Design review of the part built by this model. Coordinates are the model's own, in mm. Face numbers are marked on the shaded views. A direction names the side the tool comes from. Round coordinates to 2 decimals unless told otherwise and drop trailing zeros. Loops run counter-clockwise (first coordinate to the right, second up) from the corner with the lowest first, then second, coordinate; pieces in that order, holes last. Notation, with made-up numbers: M -23.5,25.25 L -2.5,25.25 A12 ccw -2.5,34.25 Z; hole C 86.25,80 d9. An arc over 180 degrees is marked long. One line per item, written item: value. Start each with the question number.
Item 1: For line 1 along Y through (x, z) = (-7, 2.4) (3 decimals); line 2 along Y through (x, z) = (12, 2.35); line 3 along Y through (x, z) = (-3, 2.8), list the stretches that pass through material, from the lowest coordinate up.
Item 2: For the marked faces 1, 2 and 3, list the 3-axis set-ups (+Z, -Z, +X, -X, +Y, -Y) from which the entire face can be reached by the end or side of a thin tool; tool diameter is ignored.
Item 3: Mouldability with a two-part tool opening along Y and no side actions: class the marked faces 4, 5, 6 and 7 as released by +Y, released by -Y, zero draft, split by the parting line, or undercut.
Item 4: We need section D-D (z = 2.55). State how many separate pieces and enclosed holes the cut face has, then the cut area to 3 significant figures.
Item 5: We need section A-A (x = -1.25). Write out the cut boundary in (y, z), then the cut area to 3 significant figures.
Item 6: Clearance check with flat-ended pins moving along their axes: pin 1 (1.5 mm diameter, centred on x = 2.5, z = 2, fed in from +Y); pin 2 (0.9 mm diameter, centred on y = 5, z = 1.5, fed in from -X); pin 3 (0.9 mm diameter, centred on x = -4, z = 1.5, fed in from -Y). State where each tip first meets the part, or that it passes through.
Item 7: We need section B-B (x = 11.5). Write out the cut boundary in (y, z), then the cut area to 3 significant figures.
Item 8: We need section C-C (x = -6). Write out the cut boundary in (y, z).
from build123d import *

# Parameters (mm, degrees)
BOSS_EXTRUDE1_DEPTH  = 3
SKETCH2_W            = 8
SKETCH2_H            = 3
BOSS_EXTRUDE2_DEPTH  = 7
SKETCH3_W            = 8
SKETCH3_H            = 3
BOSS_EXTRUDE3_DEPTH  = 7
SKETCH4_R            = 3.300094696
BOSS_EXTRUDE4_DEPTH  = 0.5
SKETCH5_R            = 3.300094696
BOSS_EXTRUDE5_DEPTH  = 0.5
CUT_EXTRUDE1_DEPTH   = 4
M3_CLEARANCE_HOLE2_D = 3.4
M3_CLEARANCE_HOLE1_D = 3.4
FILLET1_R            = 0.5
FILLET2_R            = 2
FILLET3_R            = 3


with BuildPart() as part:
    # Sketch1 → Boss-Extrude1 (new body)
    with BuildSketch(Plane(origin=(0, 0, 0), x_dir=(-1, 0, 0), z_dir=(0, 0, -1))):
        with BuildLine():
            Line((-16, 3), (-16, -3))
            Line((-16, -3), (9.864129683, -3))
            ThreePointArc((9.864129683, -3), (9.35323266, -6.252551424), (8.487341847, -9.429080919))
            ThreePointArc((8.487341847, -9.429080919), (3.884055388, -13.461974782), (9.996965881, -13.756600705))
            ThreePointArc((9.996965881, -13.756600705), (13.015220034, 0), (9.996965881, 13.756600705))
            ThreePointArc((9.996965881, 13.756600705), (3.884055388, 13.461974781), (8.487341847, 9.429080919))
            ThreePointArc((8.487341847, 9.429080919), (9.35323266, 6.252551424), (9.864129683, 3))
            Line((9.864129683, 3), (-16, 3))
        make_face()
    extrude(amount=-BOSS_EXTRUDE1_DEPTH)

    # Sketch2 → Boss-Extrude2 (add)
    with BuildSketch(Plane.XZ.offset(3)):
        with Locations((12, 1.5)):
            Rectangle(SKETCH2_W, SKETCH2_H)
    extrude(amount=BOSS_EXTRUDE2_DEPTH)

    # Sketch3 → Boss-Extrude3 (add)
    with BuildSketch(Plane(origin=(0, 3, 0), x_dir=(-1, 0, 0), z_dir=(0, 1, 0))):
        with Locations((-12, 1.5)):
            Rectangle(SKETCH3_W, SKETCH3_H)
    extrude(amount=BOSS_EXTRUDE3_DEPTH)

    # Sketch4 → Boss-Extrude4 (add)
    with BuildSketch(Plane.XY.offset(3)):
        with Locations((-7, 12.375)):
            Circle(SKETCH4_R)
    extrude(amount=BOSS_EXTRUDE4_DEPTH)

    # Sketch5 → Boss-Extrude5 (add)
    with BuildSketch(Plane.XY.offset(3)):
        with Locations((-7, -12.375)):
            Circle(SKETCH5_R)
    extrude(amount=BOSS_EXTRUDE5_DEPTH)

    # Sketch6 → Cut-Extrude1 (cut, through all)
    with BuildSketch(Plane.XY.offset(3)):
        with BuildLine():
            Line((8, 1.5), (-9.948163366, 1.5))
            ThreePointArc((-9.948163366, 1.5), (-9.985864188, 0), (-9.948163366, -1.5))
            Line((-9.948163366, -1.5), (8, -1.5))
            Line((8, -1.5), (8, 1.5))
        make_face()
    extrude(amount=-CUT_EXTRUDE1_DEPTH, mode=Mode.SUBTRACT)

    # M3 Clearance Hole2 (through all)
    with Locations(Plane(origin=(0, 0, 0), x_dir=(-1, 0, 0), z_dir=(0, 0, -1))):
        with Locations((-12, -7), (-12, 7)):
            Hole(M3_CLEARANCE_HOLE2_D / 2)

    # M3 Clearance Hole1 (through all)
    with Locations(Plane(origin=(0, 0, 0), x_dir=(-1, 0, 0), z_dir=(0, 0, -1))):
        with Locations((7, 12.375), (7, -12.375)):
            Hole(M3_CLEARANCE_HOLE1_D / 2)

    # Fillet1
    fillet1_edges = [part.edges().sort_by_distance(p)[0] for p in [
        (-9.864129683, 3, 1.5),
        (-9.864129683, -3, 1.5),
        (8, -3, 1.5),
        (8, 3, 1.5),
        (8, 1.5, 1.5),
        (8, -1.5, 1.5),
        (-9.948163366, -1.5, 1.5),
        (-9.948163366, 1.5, 1.5),
    ]]
    fillet(fillet1_edges, radius=FILLET1_R)

    # Fillet2
    fillet2_edges = [part.edges().sort_by_distance(p)[0] for p in [
        (-8.487341847, 9.429080919, 1.5),
        (-8.487341847, -9.429080919, 1.5),
    ]]
    fillet(fillet2_edges, radius=FILLET2_R)

    # Fillet3
    fillet3_edges = [part.edges().sort_by_distance(p)[0] for p in [
        (8, -10, 1.5),
        (16, -10, 1.5),
        (16, 10, 1.5),
        (8, 10, 1.5),
    ]]
    fillet(fillet3_edges, radius=FILLET3_R)


solid = part.part
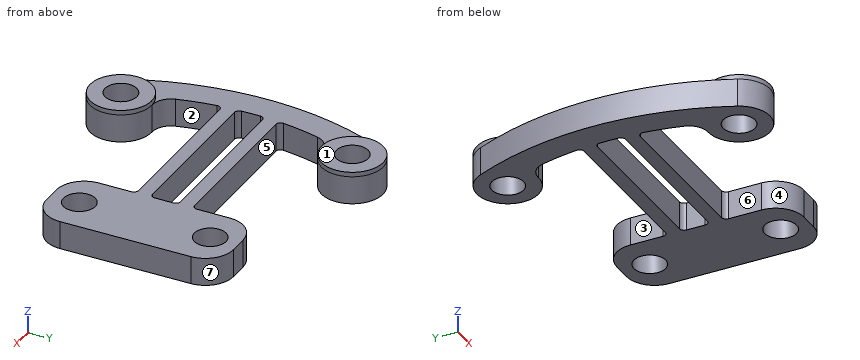
A:
1. line 1: -15.675 to -14.075, -10.675 to -9.075, -3 to -1.5, 1.5 to 3, 9.075 to 10.675, 14.075 to 15.675
1. line 2: -10 to -8.7, -5.3 to 5.3, 8.7 to 10
1. line 3: -3 to -1.5, 1.5 to 3
2. face 1: +Z, +X, -X, +Y, -Y
2. face 2: +Z, -Z
2. face 3: +Z, -Z, +Y
3. face 4: released by -Y
3. face 5: undercut
3. face 6: zero draft
3. face 7: released by +Y
4. separate pieces: 1
4. enclosed holes: 5
4. area: 306 mm2
5. outline: M -3,0 L -1.5,0 L -1.5,3 L -3,3 Z; M 1.5,0 L 3,0 L 3,3 L 1.5,3 Z
5. area: 9.00 mm2
6. pin 1: y = 3
6. pin 2: x = -12.7
6. pin 3: y = -14.47
7. outline: M -10,0 L -8.62,0 L -8.62,3 L -10,3 Z; M -5.38,0 L 5.38,0 L 5.38,3 L -5.38,3 Z; M 8.62,0 L 10,0 L 10,3 L 8.62,3 Z
7. area: 40.5 mm2
8. outline: M -15.52,0 L -13.75,0 L -13.75,3.5 L -15.52,3.5 Z; M -11,0 L -9.23,0 L -9.23,3.5 L -11,3.5 Z; M -3,0 L -1.5,0 L -1.5,3 L -3,3 Z; M 1.5,0 L 3,0 L 3,3 L 1.5,3 Z; M 9.23,0 L 11,0 L 11,3.5 L 9.23,3.5 Z; M 13.75,0 L 15.52,0 L 15.52,3.5 L 13.75,3.5 Z
